from build123d import *

# Parameters (mm, degrees)
SKETCH1_R           = 66.675
SKETCH1_R_2         = 15
BOSS_EXTRUDE1_DEPTH = 57
SKETCH2_R           = 73.025
SKETCH2_R_2         = 66.675
BOSS_EXTRUDE2_DEPTH = 9
LPATTERN1_COUNT     = 3
LPATTERN1_PITCH     = 21


with BuildPart() as part:
    # Sketch1 → Boss-Extrude1 (new body)
    with BuildSketch(Plane.XY):
        Circle(SKETCH1_R)
        Circle(SKETCH1_R_2, mode=Mode.SUBTRACT)
    extrude(amount=-BOSS_EXTRUDE1_DEPTH)

    # Sketch2 → Boss-Extrude2 (add)
    with BuildSketch(Plane.XY.offset(-3)):
        Circle(SKETCH2_R)
        Circle(SKETCH2_R_2, mode=Mode.SUBTRACT)
    boss_extrude2 = extrude(amount=-BOSS_EXTRUDE2_DEPTH)

    # LPattern1: Boss-Extrude2 ×3
    with Locations(*[(0, 0, -i * LPATTERN1_PITCH) for i in range(1, LPATTERN1_COUNT)]):
        add(boss_extrude2)


solid = part.part
Source: CAD feature listing. Evaluate the final solid. Frame: model axes, mm. A direction names the side the tool comes from. Coordinates: 2 decimals unless noted, no trailing zeros. Loops run counter-clockwise (first coordinate to the right, second up) from the corner with the lowest first, then second, coordinate; pieces in that order, holes last. Notation, with made-up numbers: (60.25, -31.75) -> (115.25, -31.75) arc R17 cw to (115.25, -21.75) -> close; hole circle Ø6 at (-18.5, -34). An arc over 180 degrees is marked (long way). Answer in a Markdown table with one row per item. Add a question column.
Q1. Pull-direction query (Z, two-part tool) for faces 1 (the face through (63.596, 20.027, -38.916)), 2 (the face through (32, -59, -3)), 3 (the face through (69.653, 21.935, -28.437)), 4 (the face through (32, -59, -54)); classes: pulls with the +Z half, pulls with the -Z half, needs draft (parallel to the pull), parting line crosses it, or undercut.
Q2. Ray query, line 1 along Z through (x, y) = (-31, -65); line 2 along Y through (x, z) = (0, -20) (3 decimals); line 3 along Y through (x, z) = (0, -27.5) (3 decimals). Return the intervals inside material, ascending.
Q3. Section C-C on z = -30. Return the cut outline in (x, y) (3 decimals).
Q4. Reachability of faces 5 (the face through (-16, 1, 0)), 6 (the face through (63.596, 20.027, -17.916)), 7 (the face through (69.653, 21.935, -49.437)), 8 (the face through (63.596, 20.027, -1.479)), 9 (the face through (63.596, 20.027, -55.479)) from +Z, -Z, +X, -X, +Y, -Y: full face, straight path, thin tool, end or side. Return the list, or none.
Q5. Contact query for flat-ended pins moving along their axis: pin 1 Ø10 at (y, z) = (-4, -36) entering from -X (3 decimals); pin 2 Ø10 at (x, z) = (55, -32) entering from -Y; pin 3 Ø5 at (y, z) = (29, -10.5) entering from -X; pin 4 Ø4 at (x, z) = (-34.5, -48) entering from -Y. Output: stop coordinate, or through.
Q6. Section D-D on x = -43.5. Return the cut outline in (y, z), and give its area (3 significant figures).
Computed values:
| question | item | result |
|---|---|---|
| 1 | face 1 | undercut |
| 1 | face 2 | pulls with the +Z half |
| 1 | face 3 | needs draft |
| 1 | face 4 | pulls with the -Z half |
| 2 | line 1 | z = -54 to -45, -33 to -24, -12 to -3 |
| 2 | line 2 | y = -66.675 to -15, 15 to 66.675 |
| 2 | line 3 | y = -73.025 to -15, 15 to 73.025 |
| 3 | outline | circle Ø146.05 at (0, 0); hole circle Ø30 at (0, 0) |
| 4 | face 5 | +Z, +X, -X, +Y, -Y |
| 4 | face 6 | none |
| 4 | face 7 | +Z, -Z |
| 4 | face 8 | +Z |
| 4 | face 9 | -Z |
| 5 | pin 1 | stops at x = -73.025 |
| 5 | pin 2 | stops at y = -53.22 |
| 5 | pin 3 | stops at x = -68.05 |
| 5 | pin 4 | stops at y = -65.39 |
| 6 | outline | (-58.65, -54) -> (-50.53, -54) -> (-50.53, -57) -> (50.53, -57) -> (50.53, -54) -> (58.65, -54) -> (58.65, -45) -> (50.53, -45) -> (50.53, -33) -> (58.65, -33) -> (58.65, -24) -> (50.53, -24) -> (50.53, -12) -> (58.65, -12) -> (58.65, -3) -> (50.53, -3) -> (50.53, 0) -> (-50.53, 0) -> (-50.53, -3) -> (-58.65, -3) -> (-58.65, -12) -> (-50.53, -12) -> (-50.53, -24) -> (-58.65, -24) -> (-58.65, -33) -> (-50.53, -33) -> (-50.53, -45) -> (-58.65, -45) -> close |
| 6 | area | 6,200 mm^2 |
